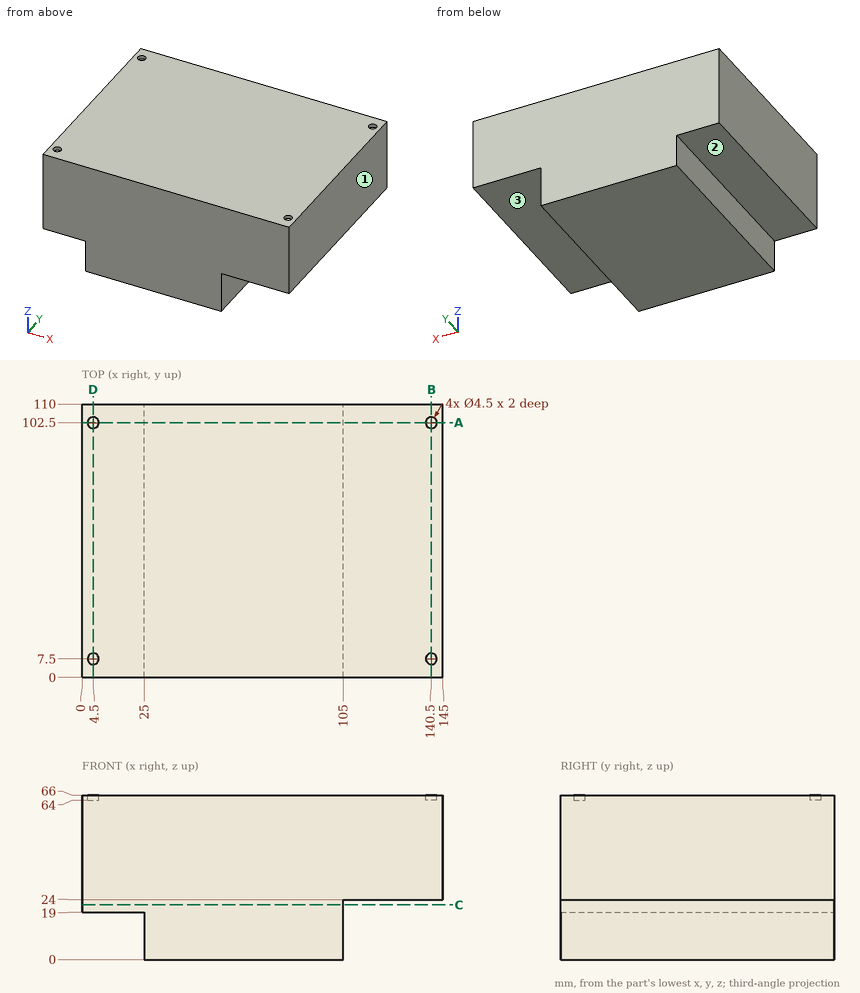
Design review of the part shown in the three views and the two pictorial views. Dimensions are in mm from the part's minimum x, y and z. A direction names the side the tool comes from. Round coordinates to 2 decimals unless told otherwise and drop trailing zeros. Loops run counter-clockwise (first coordinate to the right, second up) from the corner with the lowest first, then second, coordinate; pieces in that order, holes last. Notation, with made-up numbers: M -4.5,27.5 L 42.5,27.5 A21 cw 42.5,34.5 Z; hole C -13,67 d11. An arc over 180 degrees is marked long. Answer as a JSON object with one key per item and string values.
Item 1: We need section D-D on x = 4.5. Give the boundary of the cut face in (y, z), and give its area (3 significant figures).
Answer sheet:
{"outline": "M 0,19 L 110,19 L 110,66 L 104.75,66 L 104.75,64 L 100.25,64 L 100.25,66 L 9.75,66 L 9.75,64 L 5.25,64 L 5.25,66 L 0,66 Z", "area": "5,150 mm^2"}
Item 2: We need section A-A on y = 102.5. Give the boundary of the cut face in (x, z), and give its area (3 significant figures).
Answer sheet:
{"outline": "M 0,19 L 25,19 L 25,0 L 105,0 L 105,24 L 145,24 L 145,66 L 142.75,66 L 142.75,64 L 138.25,64 L 138.25,66 L 6.75,66 L 6.75,64 L 2.25,64 L 2.25,66 L 0,66 Z", "area": "8,120 mm^2"}
Item 3: We need section C-C on z = 22. Give the boundary of the cut face in (x, y), and give its area (4 significant figures).
Answer sheet:
{"outline": "M 0,0 L 105,0 L 105,110 L 0,110 Z", "area": "11,550 mm^2"}
Item 4: We need section B-B on x = 140.5. Give the boundary of the cut face in (y, z), and give its area (3 significant figures).
Answer sheet:
{"outline": "M 0,24 L 110,24 L 110,66 L 104.75,66 L 104.75,64 L 100.25,64 L 100.25,66 L 9.75,66 L 9.75,64 L 5.25,64 L 5.25,66 L 0,66 Z", "area": "4,600 mm^2"}
Item 5: Clearance check with flat-ended pins moving along their axes: P1, Ø10, axis at x = 118, z = 56, coming from the -Y side; P2, Ø2, axis at x = 4, y = 102, coming from the +Z side; P3, Ø1, axis at y = 32, z = 7.5, coming from the +X side; P4, Ø20, axis at x = 6.5, y = 63.5, coming from the -Z side. State where each tip first meets the part, or that it passes through.
Answer sheet:
{"P1": "stops at y = 0", "P2": "stops at z = 64", "P3": "stops at x = 105", "P4": "stops at z = 19"}
Item 6: Machinability: for the marked faces 1, 2 and 3, which of the approach directions +Z, -Z, +X, -X, +Y, -Y give a long, thin tool a straight path to every point of the face, cutting with its end or side? Answer none if there is none.
Answer sheet:
{"face 1": "+Z, -Z, +X, +Y, -Y", "face 2": "-Z, -X, +Y, -Y", "face 3": "-Z, +X, +Y, -Y"}
Item 7: Wall thickness on L1, parallel to Y at x = 4.5, z = 64.6; L2, parallel to Z at x = 121.5, y = 101; L3, parallel to X at y = 95, z = 15: over which ranges is each line inside the solid? List them lowest first. Write a range as from..to.
Answer sheet:
{"L1": "y = 0..5.25, 9.75..100.25, 104.75..110", "L2": "z = 24..66", "L3": "x = 25..105"}
